Autodesk Inventor part; units mm, degrees
ref_plane "Work Plane1" through (39.3319, 0, 0) normal (0, 0, -1) x (1, 0, 0)
ref_plane "YZ Plane" through (0, 0, 0) normal (1, 0, 0) x (0, 1, 0)
ref_plane "XZ Plane" through (0, 0, 0) normal (0, 1, 0) x (-1, 0, 0)
sketch "Эскиз1" plane through (0, 0, 0) normal (0, 0, 1) x (1, 0, 0)
  line L0 (0, 0) -> (8, 0)
  line L1 (0, 0) -> (0, 6.5)
  line L2 (8, 5.5) -> (8, 0)
  line L3 (0, 6.5) -> (8.4497, 15.0207)
  line L4 (8, 5.5) -> (13.0747, 6.6169)
  arc A0 (13.0747, 6.6169) -> (8.4497, 15.0207) centre (12, 11.5) ccw
  line L5 (8, 5.5) -> (0, 6.5)
  line L6 (8, 5.5) -> (0, 3.7393)
  dimension "d0" = 11
  dimension "d1" = 12
  dimension "d2" = 11.5
  dimension "d3" = 5
  dimension "d4" = 8
  dimension "d5" = 13
revolve "Базовый элемент" add sketch "Эскиз1" angle 360 about axis through (0, 0, 0) along (1, 0, 0) contours L1 L6 L2 L0 | L1 L5 L6
extrude "Крыло1" add sketch "Эскиз1" along normal mid plane 2.3 contours L1 L5 L6 | L5 L3 A0 L4
fillet "Сопряжение1" [suppressed]
mirror "Крыло2" about plane through (0, 0, 0) normal (0, 1, 0) of "Крыло1"
sketch "Эскиз2" plane through (0, 0, 0) normal (1, 0, 0) x (0, 1, 0)
  line L0 (0, -14) -> (0, 14)
  line L1 (-14, 0) -> (14, 0)
  point P0 (0, 0)
hole "Резьба" at (0, 0, 0) direction (1, 0, 0) diameter 4.917 end through all
chamfer "Фаска1" distance 0.5413 angle 30 1 edges at (0, 0, -2.4585) measured on face at (0, -5.0785, 0.0988)
ref_plane "Work Plane1" through (39.3319, 0, 0) normal (0, 0, -1) x (1, 0, 0)
equation "\"d0\" = KOD2"
equation "\"d1\" = KOH1 - RR"
equation "\"d2\" = 0.5 * E0 - RR"
equation "\"d3\" = RR"
equation "\"d4\" = KOH"
equation "\"d5\" = KOD"
equation "\"d6\" = SW"
equation "\"d8\" = 0.333333 * SW"
equation "\"d9\" = -0.5 * GD1 + 0.5 * NND"
equation "\"d109\" = -0.5 * GD1 + 0.5 * NND"
equation "\"NND\" = 6"
equation "\"KOH\" = 8"
equation "\"KOH1\" = 17"
equation "\"SW\" = 2.3"
equation "\"KOD\" = 13"
equation "\"KOD2\" = 11"
equation "\"RR\" = 5"
equation "\"E0\" = 33"
equation "\"GUL\" = 0.541266 * PTC"
equation "\"BOR\" = 0"
equation "\"PTC\" = 1"
equation "\"THREADDIA\" = 6"
equation "\"TOA\" = 30deg"
equation "\"RR2\" = 3"
equation "\"SW1\" = 3.3"
equation "\"GAL\" = 0.541266 * PTC"
properties part number "DIN 315 - M6" material "Сталь, мягкая"
Check sheet for the modelled part. Datum: model origin and axes. Units: mm. A direction names the side the tool comes from. Give positions to 0.01 mm unless a question says otherwise; leave off trailing zeros. Write each loop counter-clockwise with the first axis right and the second up, starting at its lowest first coordinate (ties: lowest second). Pieces come first, ordered by that corner, then holes. Notation, with made-up numbers: (15.5, 50.25) -> (36.5, 50.25) arc R10 ccw to (36.5, 68.25) -> close; hole circle Ø8 at (60.25, 73). An arc over 180 degrees is marked (long way). Use CSV: the item, a comma, the result in double quotes. Start each with the question number.
Q1. Release check for a two-part mould opening along Y. For faces 3 (the cylindrical face through (16.44, -13.8, -0.02)), 4 (the flat face through (4.284, -10.82, -0.016)), 5 (the cylindrical face through (16.32, 14.02, -0.02)), 6 (the flat face through (10, 11, 1.15)) record: +Y half, -Y half, draft (parallel to the pull), parting line (faces both ways), or undercut.
Q2. Cross-section at C-C on x = 1.25. Enter the section's corners in (y, z), and give its area (3 significant figures).
Q3. Cross-section at D-D on x = 10. Enter the section's corners in (y, z).
Q4. Tool access check on faces 1 (the cylindrical face through (4.21, -0.738, 2.345)), 2 (the flat face through (8, 1.1, -2.4)). Record the directions out of +Z, -Z, +X, -X, +Y, -Y that give a thin tool (end or side, any length) a straight path to the whole face; none if there is none.
Q5. Cross-section at B-B on y = 0. Enter the section's corners in (x, z).
Q6. Depth check by flat-ended pin: P1, Ø3.5, axis at x = 8.5, y = 13, coming from the -Z side; P2, Ø9, axis at x = 8, y = -8.5, coming from the -Z side; P3, Ø3, axis at x = 4, z = -1, coming from the +Y side. Enter the tip coordinate at first touch or a pass-through.
Q7. Cross-section at A-A on x = 12.5. Enter the section's corners in (y, z), and give its area (3 significant figures).
Q8. Scan lines: line 1 along Y through (x, z) = (4, 0); line 2 along Y through (x, z) = (13.25, -1); line 3 along X through (y, z) = (3, 2.75). Record each from-to range of solid material in increasing order.
Working result:
1,face 3,"undercut"
1,face 4,"-Y half"
1,face 5,"undercut"
1,face 6,"draft"
2,outline,"(-7.76, -1.15) -> (-6.24, -1.15) arc R6.34 ccw to (6.24, -1.15) -> (7.76, -1.15) -> (7.76, 1.15) -> (6.24, 1.15) arc R6.34 ccw to (-6.24, 1.15) -> (-7.76, 1.15) -> close; hole circle Ø4.92 at (0, 0)"
2,area,"114 mm^2"
3,outline,"(-16.08, -1.15) -> (-5.94, -1.15) -> (-5.94, 1.15) -> (-16.08, 1.15) -> close; (5.94, -1.15) -> (16.08, -1.15) -> (16.08, 1.15) -> (5.94, 1.15) -> close"
4,face 1,"+X, -X"
4,face 2,"+Z, -Z, +X"
5,outline,"(0, -6.5) -> (8, -5.5) -> (8, -2.46) -> (0.31, -2.46) -> (0, -3) -> close; (0, 3) -> (0.31, 2.46) -> (8, 2.46) -> (8, 5.5) -> (0, 6.5) -> close"
6,P1,"stops at z = -1.15"
6,P2,"stops at z = -3.84"
6,P3,"stops at y = 12.05"
7,outline,"(-16.47, -1.15) -> (-6.49, -1.15) -> (-6.49, 1.15) -> (-16.47, 1.15) -> close; (6.49, -1.15) -> (16.47, -1.15) -> (16.47, 1.15) -> (6.49, 1.15) -> close"
7,area,"45.9 mm^2"
8,line 1,"y = -10.53 to -2.46, 2.46 to 10.53"
8,line 2,"y = -16.34 to -6.66, 6.66 to 16.34"
8,line 3,"x = 0 to 8"
